Source: CAD feature listing. Evaluate the final solid. Frame: model axes, mm. Face numbers are marked on the shaded views. A direction names the side the tool comes from. Give positions to 0.01 mm unless a question says otherwise; leave off trailing zeros. Loops run counter-clockwise (first coordinate to the right, second up) from the corner with the lowest first, then second, coordinate; pieces in that order, holes last. Notation, with made-up numbers: M 66.5,14 L 109.5,14 A18 cw 109.5,43 Z; hole C -37.75,4.5 d9. An arc over 180 degrees is marked long. Write item = value, one per line.
from build123d import *

# Parameters (mm, degrees)
SKETCH2_W            = 120
SKETCH2_H            = 43
BOSS_EXTRUDE1_DEPTH  = 38
SKETCH3_W            = 116
SKETCH3_H            = 39
CUT_EXTRUDE1_DEPTH   = 38
BOSS_EXTRUDE2_DEPTH  = 39
SKETCH5_W            = 43
SKETCH5_H            = 38
BOSS_EXTRUDE3_DEPTH  = 2.5
SKETCH6_W            = 2
SKETCH6_H            = 38
BOSS_EXTRUDE4_DEPTH  = 17
SKETCH7_W            = 34
SKETCH7_H            = 38
BOSS_EXTRUDE5_DEPTH  = 10
SKETCH8_W            = 4
SKETCH8_H            = 38
BOSS_EXTRUDE6_DEPTH  = 43
SKETCH9_W            = 10
SKETCH9_H            = 5
CUT_EXTRUDE2_DEPTH   = 41
SKETCH11_W           = 120
SKETCH11_H           = 2
CUT_EXTRUDE3_DEPTH   = 110.5
CUT_EXTRUDE4_DEPTH   = 3
MIRROR4_COPY_1_DEPTH = 3
CUT_EXTRUDE5_START   = -114
SKETCH13_R           = 1
CUT_EXTRUDE5_DEPTH   = 114
SKETCH14_W           = 116
SKETCH14_H           = 2
CUT_EXTRUDE6_DEPTH   = 16.6


with BuildPart() as part:
    # Sketch2 → Boss-Extrude1 (new body)
    with BuildSketch(Plane(origin=(0, 0, 0), x_dir=(1, 0, 0), z_dir=(0, 1, 0))):
        Rectangle(SKETCH2_W, SKETCH2_H)
    extrude(amount=BOSS_EXTRUDE1_DEPTH)

    # Sketch3 → Cut-Extrude1 (cut)
    with BuildSketch(Plane(origin=(0, 38, 0), x_dir=(1, 0, 0), z_dir=(0, 1, 0))):
        Rectangle(SKETCH3_W, SKETCH3_H)
    extrude(amount=-CUT_EXTRUDE1_DEPTH, mode=Mode.SUBTRACT)

    # Sketch4 → Boss-Extrude2 (add)
    with BuildSketch(Plane.XY.offset(-19.5)):
        Polygon((-58, 0), (-58, 15), (-38, 0), align=None)
    extrude(amount=BOSS_EXTRUDE2_DEPTH)

    # Sketch5 → Boss-Extrude3 (add)
    with BuildSketch(Plane(origin=(60, 0, 0), x_dir=(0, 0, -1), z_dir=(1, 0, 0))):
        with Locations((0, 19)):
            Rectangle(SKETCH5_W, SKETCH5_H)
    extrude(amount=BOSS_EXTRUDE3_DEPTH)

    # Sketch6 → Boss-Extrude4 (add)
    with BuildSketch(Plane(origin=(0, 0, -21.5), x_dir=(-1, 0, 0), z_dir=(0, 0, -1))):
        with Locations((-61.5, 19)):
            Rectangle(SKETCH6_W, SKETCH6_H)
    extrude(amount=BOSS_EXTRUDE4_DEPTH)

    # Mirror1: part across plane


with BuildPart() as part_1:
    add(part.part)
    add(part.part.mirror(Plane(origin=(0, 0, -38.5), x_dir=(1, 0, 0), z_dir=(0, 0, -1))))

    # Sketch7 → Boss-Extrude5 (add)
    with BuildSketch(Plane(origin=(62.5, 0, 0), x_dir=(0, 0, -1), z_dir=(1, 0, 0))):
        with Locations((38.5, 19)):
            Rectangle(SKETCH7_W, SKETCH7_H)
    extrude(amount=BOSS_EXTRUDE5_DEPTH)

    # Sketch8 → Boss-Extrude6 (add)
    with BuildSketch(Plane.XY.offset(-21.5)):
        with Locations((70.5, 19)):
            Rectangle(SKETCH8_W, SKETCH8_H)
    boss_extrude6 = extrude(amount=BOSS_EXTRUDE6_DEPTH)

    # Sketch9 → Cut-Extrude2 (cut)
    with BuildSketch(Plane.XY.offset(21.5)):
        with Locations((65.5, 27.5)):
            Rectangle(SKETCH9_W, SKETCH9_H)
        with Locations((65.5, 10.5)):
            Rectangle(SKETCH9_W, SKETCH9_H)
    cut_extrude2 = extrude(amount=-CUT_EXTRUDE2_DEPTH, mode=Mode.SUBTRACT)

    # Mirror2: Boss-Extrude6, Cut-Extrude2 across plane
    add(boss_extrude6.mirror(Plane(origin=(0, 0, -38.5), x_dir=(1, 0, 0), z_dir=(0, 0, -1))))
    add(cut_extrude2.mirror(Plane(origin=(0, 0, -38.5), x_dir=(1, 0, 0), z_dir=(0, 0, -1))), mode=Mode.SUBTRACT)

    # Sketch11 → Cut-Extrude3 (cut)
    with BuildSketch(Plane(origin=(72.5, 0, 0), x_dir=(0, 0, -1), z_dir=(1, 0, 0))):
        with Locations((38.5, 1)):
            Rectangle(SKETCH11_W, SKETCH11_H)
    extrude(amount=-CUT_EXTRUDE3_DEPTH, mode=Mode.SUBTRACT)

    # Sketch12 → Cut-Extrude4 (cut)
    with BuildSketch(Plane.XY.offset(21.5)):
        with BuildLine():
            Line((-38, 2), (-49.614835193, 2))
            ThreePointArc((-49.614835193, 2), (-56.018375168, 7.287996976), (-60, 0))
            Line((-60, 0), (-38, 0))
            Line((-38, 0), (-38, 2))
        make_face()
    cut_extrude4 = extrude(amount=-CUT_EXTRUDE4_DEPTH, mode=Mode.SUBTRACT)

    # Mirror3: Cut-Extrude4 across plane
    add(cut_extrude4.mirror(Plane.XY), mode=Mode.SUBTRACT)

    # Mirror4: Cut-Extrude4 across plane
    add(cut_extrude4.mirror(Plane(origin=(0, 0, -38.5), x_dir=(1, 0, 0), z_dir=(0, 0, -1))), mode=Mode.SUBTRACT)

    # Mirror4 copy 1 sketch → Mirror4 copy 1 (cut)
    with BuildSketch(Plane.XY.offset(-55.5)):
        with BuildLine():
            Line((-38, 2), (-49.614835193, 2))
            ThreePointArc((-49.614835193, 2), (-56.018375168, 7.287996976), (-60, 0))
            Line((-60, 0), (-38, 0))
            Line((-38, 0), (-38, 2))
        make_face()
    extrude(amount=-MIRROR4_COPY_1_DEPTH, mode=Mode.SUBTRACT)

    # Sketch13 → Cut-Extrude5 (cut)
    with BuildSketch(Plane.XY.offset(18.5).offset(CUT_EXTRUDE5_START)):
        with Locations((-58, 2)):
            Circle(SKETCH13_R)
    extrude(amount=CUT_EXTRUDE5_DEPTH, mode=Mode.SUBTRACT)

    # Chamfer1
    # the kernel refuses this chamfer: 10 mm, written as the material it takes off along each edge
    with BuildSketch(Plane(origin=(-49.614835193, 2, 38.180669666), x_dir=(-0.41152080336556635, 0.9114003666870882, 0), z_dir=(0, 0, -1))) as chamfer1_piece_1:
        with BuildLine():
            Line((4.024103798, 0), (-2.897424879, 6.010331734))
            Line((-2.897424879, 6.010331734), (-3.079704953, 5.928027573))
            ThreePointArc((-3.079704953, 5.928027573), (-1.554736759, 2.957293148), (-0.182280073, -0.082304161))
            Line((-0.182280073, -0.082304161), (0.082304161, -0.182280073))
            ThreePointArc((0.082304161, -0.182280073), (2.000716354, 0.27264804), (3.968173362, -0.192020276))
            Line((3.968173362, -0.192020276), (4.024103798, 0))
        make_face()
    extrude(amount=19.680669666, mode=Mode.SUBTRACT)

    # Chamfer2
    # the kernel refuses this chamfer: 10 mm, written as the material it takes off along each edge
    with BuildSketch(Plane(origin=(-49.614835193, 2, -38.180669666), x_dir=(0.9996854583228201, -0.0250795617564035, 0), z_dir=(0, 0, 1))) as chamfer2_piece_1:
        with BuildLine():
            Line((6.672267866, 0), (-1.747462586, 3.624884258))
            Line((-1.747462586, 3.624884258), (-1.896145364, 3.491117927))
            ThreePointArc((-1.896145364, 3.491117927), (-0.623209418, 1.920628258), (-0.199937092, -0.005015912))
            Line((-0.199937092, -0.005015912), (0.005015912, -0.199937092))
            ThreePointArc((0.005015912, -0.199937092), (3.339051469, -0.116294632), (6.677283779, -0.199937092))
            Line((6.677283779, -0.199937092), (6.672267866, 0))
        make_face()
    extrude(amount=19.680669666, mode=Mode.SUBTRACT)

    # Chamfer3
    # the kernel refuses this chamfer: 10 mm, written as the material it takes off along each edge
    with BuildSketch(Plane(origin=(-49.614835193, 2, -38.819330334), x_dir=(0.9996854583228201, -0.02507956175640344, 0), z_dir=(0, 0, -1))) as chamfer3_piece_1:
        with BuildLine():
            Line((6.672267866, 0), (-1.747462586, -3.624884258))
            Line((-1.747462586, -3.624884258), (-1.896145364, -3.491117927))
            ThreePointArc((-1.896145364, -3.491117927), (-0.623209418, -1.920628258), (-0.199937092, 0.005015912))
            Line((-0.199937092, 0.005015912), (0.005015912, 0.199937092))
            ThreePointArc((0.005015912, 0.199937092), (3.339051469, 0.116294632), (6.677283779, 0.199937092))
            Line((6.677283779, 0.199937092), (6.672267866, 0))
        make_face()
    extrude(amount=19.680669666, mode=Mode.SUBTRACT)

    # Chamfer4
    # the kernel refuses this chamfer: 10 mm, written as the material it takes off along each edge
    with BuildSketch(Plane(origin=(-49.614835193, 2, -115.180669666), x_dir=(0.9996854583228201, -0.0250795617564035, 0), z_dir=(0, 0, 1))) as chamfer4_piece_1:
        with BuildLine():
            Line((6.672267866, 0), (-1.747462586, 3.624884258))
            Line((-1.747462586, 3.624884258), (-1.896145364, 3.491117927))
            ThreePointArc((-1.896145364, 3.491117927), (-0.623209418, 1.920628258), (-0.199937092, -0.005015912))
            Line((-0.199937092, -0.005015912), (0.005015912, -0.199937092))
            ThreePointArc((0.005015912, -0.199937092), (3.339051469, -0.116294632), (6.677283779, -0.199937092))
            Line((6.677283779, -0.199937092), (6.672267866, 0))
        make_face()
    extrude(amount=19.680669666, mode=Mode.SUBTRACT)

    # Sketch14 → Cut-Extrude6 (cut)
    with BuildSketch(Plane(origin=(0, 38, 0), x_dir=(1, 0, 0), z_dir=(0, 1, 0))):
        with Locations((0, 20.5)):
            Rectangle(SKETCH14_W, SKETCH14_H)
    cut_extrude6 = extrude(amount=-CUT_EXTRUDE6_DEPTH, mode=Mode.SUBTRACT)

    # Mirror5: Cut-Extrude6 across plane
    add(cut_extrude6.mirror(Plane(origin=(0, 0, -38.5), x_dir=(1, 0, 0), z_dir=(0, 0, -1))), mode=Mode.SUBTRACT)


solid = part_1.part
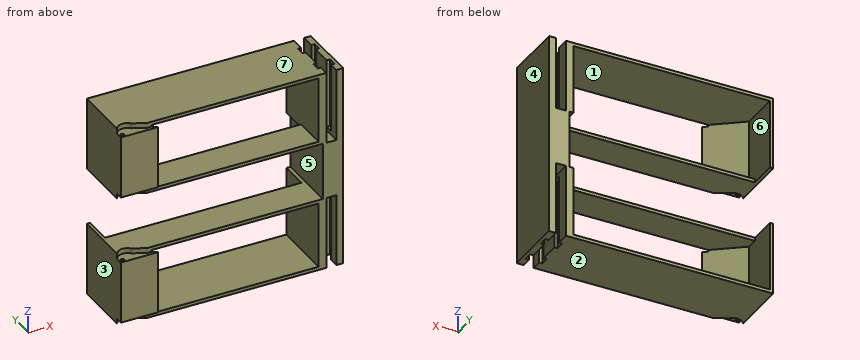
1. Reachability of the marked faces 5, 6 and 7 from +Z, -Z, +X, -X, +Y, -Y: full face, straight path, thin tool, end or side. Return the list, or none.
Derived:
face_5 = -X, +Y, -Y
face_6 = +Y
face_7 = +Z, +X, -X, +Y, -Y
2. Cut plane B-B, the plane x = -17.5. Return the cut outline in (y, z).
Derived:
outline = M 2,-98.5 L 38,-98.5 L 38,-96.5 L 2,-96.5 Z; M 2,-57.5 L 21.4,-57.5 L 21.4,-55.5 L 2,-55.5 Z; M 2,-21.5 L 21.4,-21.5 L 21.4,-19.5 L 2,-19.5 Z; M 2,19.5 L 38,19.5 L 38,21.5 L 2,21.5 Z
3. Cut plane C-C, the plane y = 18. Return the cut outline in (x, z), then the cut area to 3 significant figures.
Derived:
outline = M -60,-98.5 L 62.5,-98.5 L 62.5,-55.5 L 68.5,-55.5 L 68.5,-98.5 L 72.5,-98.5 L 72.5,21.5 L 68.5,21.5 L 68.5,-21.5 L 62.5,-21.5 L 62.5,21.5 L -60,21.5 L -60,-21.5 L 60.5,-21.5 L 60.5,-55.5 L -60,-55.5 Z; hole M -58,-96.5 L 58,-96.5 L 58,-57.5 L -58,-57.5 Z; hole M -58,-19.5 L 58,-19.5 L 58,19.5 L -58,19.5 Z
area = 2,240 mm²
4. First-contact query: pin 1 Ø1.8 at (x, y) = (66.5, 12) entering from +Z; pin 2 Ø0.6 at (x, y) = (61.5, 27) entering from +Z; pin 3 Ø1.6 at (x, z) = (61.5, -0.5) entering from -Y. Flat tips, straight axial feed; report the tip coordinate or a pass-through.
Derived:
pin_1 = -21.5
pin_2 = -19.5
pin_3 = 2
5. Cut plane A-A, the plane z = -15.5. Count the separate pieces of the cut face and the enclosed holes in it, then the cut area to 3 significant figures.
Derived:
separate_pieces = 3
enclosed_holes = 1
area = 489 mm²
6. Material intervals for probe 1 along X at (y, z) = (28.5, -18); probe 2 along Z at (x, y) = (-25, 5); probe 3 along X at (y, z) = (34.5, -6), sorted ascending. Write a range as from..to.
Derived:
probe_1 = -60..-58, 58..60.5, 70.5..72.5
probe_2 = -98.5..-96.5, -57.5..-55.5, -21.5..-19.5, 19.5..21.5
probe_3 = -60..-58, 58..62.5, 68.5..72.5
7. Pull-direction query (X, two-part tool) for the marked faces 1, 2, 3 and 4; classes: +X half, -X half, draft (parallel to the pull), parting line (faces both ways), or undercut.
Derived:
face_1 = undercut
face_2 = draft
face_3 = -X half
face_4 = +X half
